```python
from build123d import *

# Parameters (mm, degrees)
BOSS_EXTRUDE1_DEPTH                      = 58.7375
SKETCH2_R                                = 20.066
BOSS_EXTRUDE2_DEPTH                      = 73.66
EDIT_LENGTH_HERE_HOVER_FOR_COMMENT_DEPTH = 113.792
SKETCH4_R                                = 9.9822
BOSS_EXTRUDE4_DEPTH                      = 19.05
BOSS_EXTRUDE5_DEPTH                      = 20.6502
CUT_EXTRUDE3_DEPTH                       = 211.434564151
CUT_EXTRUDE3_DEPTH_BACK                  = 211.434564151
SKETCH6_R                                = 3.3782
FILLET1_R                                = 2.54
FILLET2_R                                = 0.508
CUT_EXTRUDE5_DEPTH                       = 3.81
SKETCH8_R                                = 6.5405
BOSS_EXTRUDE6_DEPTH                      = 4.445
FILLET3_R                                = 0.0254
BOSS_EXTRUDE7_START                      = -12.7
BOSS_EXTRUDE7_DEPTH                      = 12.7
SKETCH10_R                               = 2.54
BOSS_EXTRUDE8_DEPTH                      = 0.635


with BuildPart() as part:
    # Sketch1 → Boss-Extrude1 (new body)
    with BuildSketch(Plane.XY):
        with BuildLine():
            Line((-12.7, 0), (12.7, 0))
            Line((12.7, 0), (20.955, 6.35))
            Line((20.955, 6.35), (20.955, 60.833))
            ThreePointArc((20.955, 60.833), (0, 81.788), (-20.955, 60.833))
            Line((-20.955, 60.833), (-20.955, 6.35))
            Line((-20.955, 6.35), (-12.7, 0))
        make_face()
    extrude(amount=BOSS_EXTRUDE1_DEPTH)

    # Sketch2 → Boss-Extrude2 (add)
    with BuildSketch(Plane.XY.offset(58.7375)):
        with Locations(Location((0, 60.833, 0), (0, 0, 180))):
            Circle(SKETCH2_R)
    extrude(amount=BOSS_EXTRUDE2_DEPTH)

    # Sketch3 → EDIT_LENGTH_HERE (hover for comment) (add)
    with BuildSketch(Plane.XY.offset(58.7375)):
        with BuildLine():
            Line((-14.88814822, 20.042680112), (-10.996912775, 1.5621))
            Line((-10.996912775, 1.5621), (10.996912775, 1.5621))
            Line((10.996912775, 1.5621), (14.88814822, 20.042680112))
            ThreePointArc((14.88814822, 20.042680112), (0, 38.3921), (-14.88814822, 20.042680112))
        make_face()
    extrude(amount=EDIT_LENGTH_HERE_HOVER_FOR_COMMENT_DEPTH)

    # Sketch4 → Boss-Extrude4 (add)
    with BuildSketch(Plane.XY.offset(172.5295)):
        with Locations(Location((0, 23.1775, 0), (0, 0, 180))):
            Circle(SKETCH4_R)
    extrude(amount=BOSS_EXTRUDE4_DEPTH)

    # Sketch5 → Boss-Extrude5 (add)
    with BuildSketch(Plane(origin=(0, 0, 0), x_dir=(-1, 0, 0), z_dir=(0, 0, -1))):
        with BuildLine():
            Line((-3.81, 32.0675), (3.81, 32.0675))
            ThreePointArc((3.81, 32.0675), (7.402102448, 30.579602448), (8.89, 26.9875))
            Line((8.89, 26.9875), (8.89, 19.3675))
            ThreePointArc((8.89, 19.3675), (7.402102448, 15.775397552), (3.81, 14.2875))
            Line((3.81, 14.2875), (-3.81, 14.2875))
            ThreePointArc((-3.81, 14.2875), (-7.402102448, 15.775397552), (-8.89, 19.3675))
            Line((-8.89, 19.3675), (-8.89, 26.9875))
            ThreePointArc((-8.89, 26.9875), (-7.402102448, 30.579602448), (-3.81, 32.0675))
        make_face()
    extrude(amount=BOSS_EXTRUDE5_DEPTH)

    # Sketch6 → Cut-Extrude3 (cut, two sides: drawn at the far end of the back side and taken through both)
    with BuildSketch(Plane(origin=(8.89, 0, 0), x_dir=(0, 0, -1), z_dir=(1, 0, 0)).offset(-CUT_EXTRUDE3_DEPTH_BACK)):
        with Locations((11.90625, 23.1775)):
            Circle(SKETCH6_R)
        with Locations(Location((-182.0545, 23.1775, 0), (0, 0, 179.999999986))):
            Circle(SKETCH6_R)
    extrude(amount=CUT_EXTRUDE3_DEPTH + CUT_EXTRUDE3_DEPTH_BACK, mode=Mode.SUBTRACT)

    # Fillet1
    fillet1_edges = [part.edges().sort_by_distance(p)[0] for p in [
        (7.402102448, 15.775397552, 0),
        (0, 14.2875, 0),
        (-7.402102448, 15.775397552, 0),
        (-8.89, 23.1775, 0),
        (-7.402102448, 30.579602448, 0),
        (0, 32.0675, 0),
        (7.402102448, 30.579602448, 0),
        (8.89, 23.1775, 0),
    ]]
    fillet(fillet1_edges, radius=FILLET1_R)

    # Fillet2
    fillet2_edges = [part.edges().sort_by_distance(p)[0] for p in [
        (7.402102448, 15.775397552, -20.6502),
        (0, 14.2875, -20.6502),
        (-7.402102448, 15.775397552, -20.6502),
        (-8.89, 23.1775, -20.6502),
        (-7.402102448, 30.579602448, -20.6502),
        (0, 32.0675, -20.6502),
        (7.402102448, 30.579602448, -20.6502),
        (8.89, 23.1775, -20.6502),
    ]]
    fillet(fillet2_edges, radius=FILLET2_R)

    # Sketch7 → Cut-Extrude5 (cut)
    with BuildSketch(Plane(origin=(0, 0, 0), x_dir=(-1, 0, 0), z_dir=(0, 0, -1))):
        with BuildLine():
            Line((-4.1275, 80.068311519), (-4.1275, 77.089))
            ThreePointArc((-4.1275, 77.089), (0, 72.9615), (4.1275, 77.089))
            Line((4.1275, 77.089), (4.1275, 79.978628931))
            ThreePointArc((4.1275, 79.978628931), (4.367379625, 80.721429048), (4.996400809, 81.183626623))
            ThreePointArc((4.996400809, 81.183626623), (0.071861599, 81.787876781), (-4.856706104, 81.217416372))
            ThreePointArc((-4.856706104, 81.217416372), (-4.325187488, 80.748786262), (-4.1275, 80.068311519))
        make_face()
        with BuildLine():
            ThreePointArc((-19.685, 11.610879552), (-20.583025612, 11.98285394), (-20.955, 12.880879552))
            Line((-20.955, 12.880879552), (-20.955, 6.35))
            Line((-20.955, 6.35), (-13.042377801, 0.26336754))
            ThreePointArc((-13.042377801, 0.26336754), (-13.507857108, 0.994743297), (-13.395607029, 1.854383572))
            Line((-13.395607029, 1.854383572), (-11.222314297, 6.047728836))
            ThreePointArc((-11.222314297, 6.047728836), (-11.349573436, 9.780348644), (-14.605, 11.610879552))
            Line((-14.605, 11.610879552), (-19.685, 11.610879552))
        make_face()
        with BuildLine():
            Line((20.955, 6.35), (20.955, 12.880879552))
            ThreePointArc((20.955, 12.880879552), (20.583025612, 11.98285394), (19.685, 11.610879552))
            Line((19.685, 11.610879552), (14.605, 11.610879552))
            ThreePointArc((14.605, 11.610879552), (11.203032914, 9.51631534), (11.541558483, 5.535614431))
            Line((11.541558483, 5.535614431), (13.402295436, 1.841293477))
            ThreePointArc((13.402295436, 1.841293477), (13.506243345, 0.987572709), (13.042377827, 0.263367559))
            Line((13.042377827, 0.263367559), (20.955, 6.35))
        make_face()
    extrude(amount=-CUT_EXTRUDE5_DEPTH, mode=Mode.SUBTRACT)

    # Sketch8 → Boss-Extrude6 (add)
    with BuildSketch(Plane.XY.offset(132.3975)):
        with Locations((0, 60.833)):
            Circle(SKETCH8_R)
    extrude(amount=BOSS_EXTRUDE6_DEPTH)

    # Fillet3
    fillet3_edges = [part.edges().sort_by_distance(p)[0] for p in [
        (-6.5405, 60.833, 132.3975),
        (-6.5405, 60.833, 136.8425),
    ]]
    fillet(fillet3_edges, radius=FILLET3_R)

    # Sketch9 → Boss-Extrude7 (add)
    with BuildSketch(Plane.XY.offset(172.5295).offset(BOSS_EXTRUDE7_START)):
        with BuildLine():
            Line((-11.017521545, 1.5367), (11.017521545, 1.5367))
            Line((11.017521545, 1.5367), (14.913003226, 20.03744669))
            ThreePointArc((14.913003226, 20.03744669), (0, 38.4175), (-14.913003226, 20.03744669))
            Line((-14.913003226, 20.03744669), (-11.017521545, 1.5367))
        make_face()
        with BuildLine():
            Line((10.996912775, 1.5621), (14.88814822, 20.042680112))
            ThreePointArc((14.88814822, 20.042680112), (0, 38.3921), (-14.88814822, 20.042680112))
            Line((-14.88814822, 20.042680112), (-10.996912775, 1.5621))
            Line((-10.996912775, 1.5621), (10.996912775, 1.5621))
        make_face(mode=Mode.SUBTRACT)
    extrude(amount=BOSS_EXTRUDE7_DEPTH)

    # Sketch10 → Boss-Extrude8 (add)
    with BuildSketch(Plane(origin=(0, 0, 3.81), x_dir=(-1, 0, 0), z_dir=(0, 0, -1))):
        with Locations((0, 77.089)):
            Circle(SKETCH10_R)
        with Locations((-14.605, 7.800879552)):
            Circle(SKETCH10_R)
        with Locations((14.605, 7.800879552)):
            Circle(SKETCH10_R)
    extrude(amount=BOSS_EXTRUDE8_DEPTH)


solid = part.part
```
Input: part model. Units: mm. Frame: model coordinates. A direction names the side the tool comes from. Coordinates: 2 decimals unless noted, no trailing zeros. Loops run counter-clockwise (first coordinate to the right, second up) from the corner with the lowest first, then second, coordinate; pieces in that order, holes last. Notation, with made-up numbers: M 63.5,52 L 67.5,52 A11 cw 67.5,59 Z; hole C -8.75,44 d1. An arc over 180 degrees is marked long. Answer in a Markdown table with one row per item.
1. Material intervals for line 1 (Z direction, x = -7, y = 22); line 2 (Y direction, x = 5, z = 43.5); line 3 (Z direction, x = 13.5, y = 14), sorted ascending.
Response:
| item | result |
|---|---|
| line 1 | z = -20.65 to -15.07, -8.74 to 178.89, 185.22 to 191.58 |
| line 2 | y = 0 to 81.18 |
| line 3 | z = 0 to 172.53 |
2. Section A-A, the plane z = 116. Output: boundary loops of the cut face in (x, y), then the cut area to 3 significant figures.
Response:
| item | result |
|---|---|
| outline | C 0,60.83 d40.13; M -14.89,20.04 L -11,1.56 L 11,1.56 L 14.89,20.04 A15.21 ccw long Z |
| area | 2,200 mm2 |
3. First-contact query: pin 1 (8.5 mm diameter, centred on x = 1, z = -13.5, fed in from -Y); pin 2 (5.5 mm diameter, centred on x = 14, y = 6.5, fed in from -Z); pin 3 (8 mm diameter, centred on y = 23.18, z = -11.91, fed in from -X). Flat tips, straight axial feed; report the tip coordinate or a pass-through.
Response:
| item | result |
|---|---|
| pin 1 | stops at y = 14.29 |
| pin 2 | stops at z = 0 |
| pin 3 | stops at x = -8.89 |
4. Section D-D, the plane x = 0. Count the separate pieces of the cut face and the enclosed holes in it, then the cut area to 3 significant figures.
Response:
| item | result |
|---|---|
| separate pieces | 1 |
| enclosed holes | 2 |
| area | 12,700 mm2 |
5. Draft query along Y for faces 1 (the flat face through (12.915, 10.673, 108.576)), 2 (the flat face through (-15, 8, 3.175)), 3 (the flat face through (0, 77, 3.175)). Return one class per face: pulls with the +Y half, pulls with the -Y half, needs draft (parallel to the pull), parting line crosses it, or undercut.
Response:
| item | result |
|---|---|
| face 1 | pulls with the -Y half |
| face 2 | undercut |
| face 3 | needs draft |
6. Section B-B, the plane y = 51. Output: boundary loops of the cut face in (x, z) (1 decimal).
Response:
| item | result |
|---|---|
| outline | M -21,0 L 21,0 L 21,58.7 L 17.5,58.7 L 17.5,132.4 L -17.5,132.4 L -17.5,58.7 L -21,58.7 Z |
7. Reachability of faces 4 (the cylindrical face through (15.156, 5.321, 3.497)), 5 (the cylindrical face through (7.44, 30.54, -11.22)), 6 (the cylindrical face through (-7.441, 15.815, -11.218)), 7 (the cylindrical face through (2.612, 40.938, 95.052)), 8 (the flat face through (15, 8, 3.175)) from +Z, -Z, +X, -X, +Y, -Y: full face, straight path, thin tool, end or side. Return the list, or none.
Response:
| item | result |
|---|---|
| face 4 | -Z |
| face 5 | -Z, +X, +Y |
| face 6 | -Z, -X, -Y |
| face 7 | +Z |
| face 8 | -Z, +X |
8. Section C-C, the plane z = 11.5. Output: boundary loops of the cut face in (x, y) (3 decimals).
Response:
| item | result |
|---|---|
| outline | M -20.955,6.35 L -12.7,0 L 12.7,0 L 20.955,6.35 L 20.955,60.833 A20.955 ccw -20.955,60.833 Z |
